from build123d import *

# Parameters (mm, degrees)
SKETCH1_W           = 310.63946
SKETCH1_H           = 92.869200088
BOSS_EXTRUDE1_DEPTH = 143.6878
SKETCH2_R           = 6.35
CUT_EXTRUDE1_DEPTH  = 144.6878
SKETCH3_W           = 310.82742
SKETCH3_H           = 12.7
CUT_EXTRUDE2_DEPTH  = 25.4
SKETCH4_W           = 25.653918198
SKETCH4_H           = 4.153491518
CUT_EXTRUDE3_DEPTH  = 2.54


with BuildPart() as part:
    # Sketch1 → Boss-Extrude1 (new body)
    with BuildSketch(Plane(origin=(0, 0, 0), x_dir=(1, 0, 0), z_dir=(0, 1, 0))):
        with Locations((155.31973, 46.434600044)):
            Rectangle(SKETCH1_W, SKETCH1_H)
    extrude(amount=BOSS_EXTRUDE1_DEPTH)

    # Sketch2 → Cut-Extrude1 (cut, through all)
    with BuildSketch(Plane(origin=(0, 143.6878, 0), x_dir=(1, 0, 0), z_dir=(0, 1, 0))):
        with Locations((46.5328, 46.14164)):
            Circle(SKETCH2_R)
        with Locations((264.10666, 46.14164)):
            Circle(SKETCH2_R)
    extrude(amount=-CUT_EXTRUDE1_DEPTH, mode=Mode.SUBTRACT)

    # Sketch3 → Cut-Extrude2 (cut)
    with BuildSketch(Plane(origin=(0, 143.6878, 0), x_dir=(1, 0, 0), z_dir=(0, 1, 0))):
        with Locations((155.41371, 87.68842)):
            Rectangle(SKETCH3_W, SKETCH3_H)
    cut_extrude2 = extrude(amount=-CUT_EXTRUDE2_DEPTH, mode=Mode.SUBTRACT)

    # Mirror1: Cut-Extrude2 across plane
    add(cut_extrude2.mirror(Plane.ZX.offset(71.8439)), mode=Mode.SUBTRACT)

    # Sketch4 → Cut-Extrude3 (cut)
    with BuildSketch(Plane(origin=(0, 143.6878, 0), x_dir=(1, 0, 0), z_dir=(0, 1, 0))):
        Polygon((43.786266597, 21.391489422), (43.786266597, 8.564530323), (47.695435084, 8.564530323), (47.695435084, 21.391489422), (61.62184782, 21.391489422), (61.62184782, 23.956881242), (47.695435084, 23.956881242), (47.695435084, 34.218448521), (43.786266597, 34.218448521), (43.786266597, 23.956881242), (30.837145982, 23.956881242), (30.837145982, 21.391489422), align=None)
        with Locations((265.020770675, 21.880135483)):
            Rectangle(SKETCH4_W, SKETCH4_H)
    extrude(amount=-CUT_EXTRUDE3_DEPTH, mode=Mode.SUBTRACT)


solid = part.part
Read the model definition and answer for the solid it produces. Units are mm, in the model's axes. A direction names the side the tool comes from. Coordinates: 2 decimals unless noted, no trailing zeros. Order: outer loops, then holes, each group sorted by start corner. A loop starts at its lowest first (then second) coordinate and runs counter-clockwise, first axis right, second up. Notation, with made-up numbers: (26.25, -40) -> (37.25, -40) arc R14 ccw to (37.25, -21) -> close; hole circle Ø8 at (61.25, 19.5). An arc over 180 degrees is marked (long way). Answer as a JSON object with one key per item and string values.
1) Each of these flat-tipped pins is pushed along its axis until it touches: pin 1 (1.3 mm diameter, centred on y = 142, z = -16, fed in from -X); pin 2 (2 mm diameter, centred on x = 56.5, y = 142.5, fed in from -Z); pin 3 (12.5 mm diameter, centred on x = 188.5, z = -89.5, fed in from -Y). Where does it stop, or does it pass through?
Model answer:
{"pin 1": "stops at x = 0", "pin 2": "stops at z = -81.34", "pin 3": "stops at y = 25.4"}
2) A cutting plane is placed at A-A, the plane x = 275. Determine the outline of the cut face in (y, z).
Model answer:
{"outline": "(0, -81.34) -> (25.4, -81.34) -> (25.4, -92.87) -> (118.29, -92.87) -> (118.29, -81.34) -> (143.69, -81.34) -> (143.69, -23.96) -> (141.15, -23.96) -> (141.15, -19.8) -> (143.69, -19.8) -> (143.69, 0) -> (0, 0) -> close"}
3) Consider line 1 along Z through (x, y) = (71.5, 12); line 2 along Z through (x, y) = (264, 18.5); line 3 along X through (y, z) = (82, -52). Determine where each line is inside the solid, lowest interval first. Write a range as from..to.
Model answer:
{"line 1": "z = -81.34..0", "line 2": "z = -81.34..-52.49, -39.79..0", "line 3": "x = 0..44.08, 48.98..261.66, 266.56..310.64"}
4) The mould has two halves that part along X. Classify faces 1 (the face through (310.639, 71, -46)), 2 (the face through (0, 71, -46)), 3 (the face through (153, 71, 0)), 4 (the face through (46, 141.148, -21)): released by +X, released by -X, zero draft, split by the parting line, or undercut.
Model answer:
{"face 1": "released by +X", "face 2": "released by -X", "face 3": "zero draft", "face 4": "undercut"}
5) A cutting plane is placed at C-C, the plane z = -86. Determine the outline of the cut face in (x, y), plus the area to 3 significant figures.
Model answer:
{"outline": "(0, 25.4) -> (310.64, 25.4) -> (310.64, 118.29) -> (0, 118.29) -> close", "area": "28,900 mm²"}
6) A cutting plane is placed at D-D, the plane x = 99. Determine the outline of the cut face in (y, z), plus the area to 3 significant figures.
Model answer:
{"outline": "(0, -81.34) -> (25.4, -81.34) -> (25.4, -92.87) -> (118.29, -92.87) -> (118.29, -81.34) -> (143.69, -81.34) -> (143.69, 0) -> (0, 0) -> close", "area": "12,800 mm²"}
7) A tool of negligible diameter and unlimited length cuts with its end or side. For faces 5 (the face through (153, 118.288, -87)), 6 (the face through (153, 25.4, -87)), 7 (the face through (41.85, 72.85, -50.43)), from which of +Z, -Z, +X, -X, +Y, -Y can it reach the whole face along a straight path? Write none if from no direction.
Model answer:
{"face 5": "-Z, +X, -X, +Y", "face 6": "-Z, +X, -X, -Y", "face 7": "+Y, -Y"}
8) A cutting plane is placed at B-B, the plane y = 19. Determine the outline of the cut face in (x, z).
Model answer:
{"outline": "(0, -81.34) -> (310.64, -81.34) -> (310.64, 0) -> (0, 0) -> close; hole circle Ø12.7 at (46.53, -46.14); hole circle Ø12.7 at (264.11, -46.14)"}
